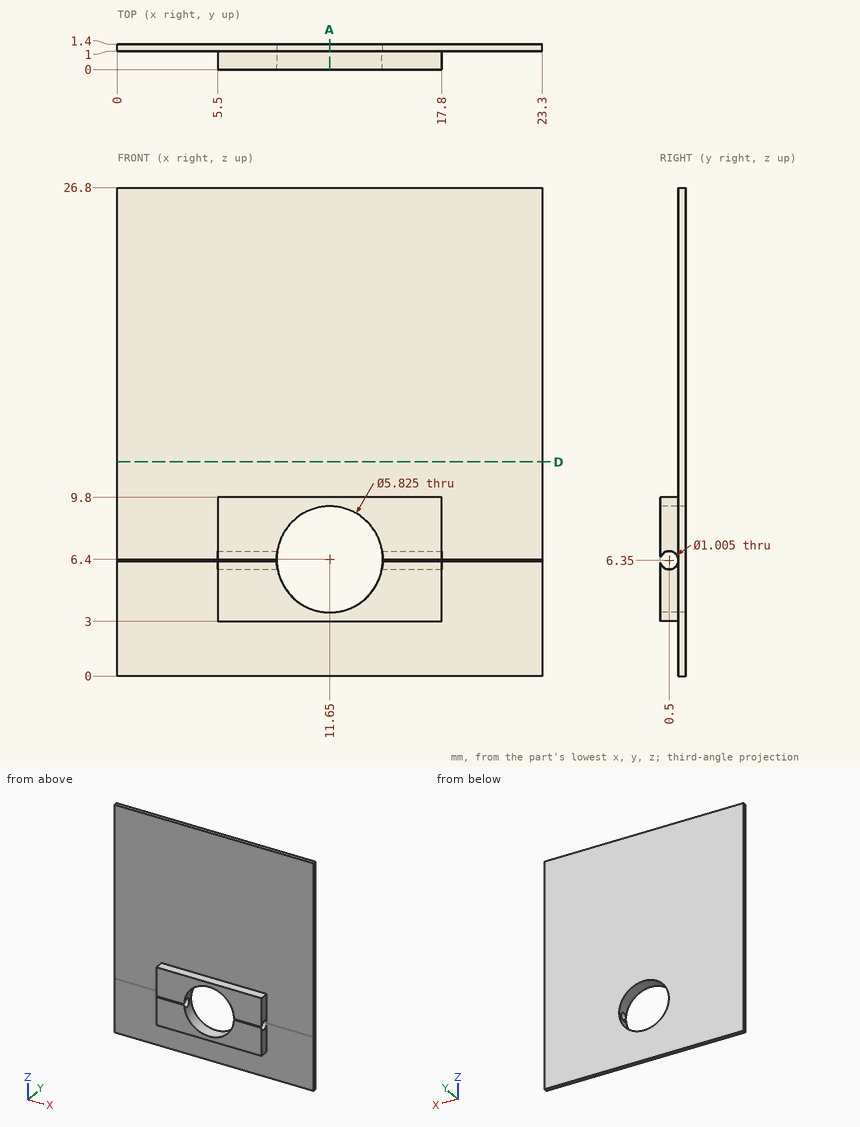
Print and shaded views of the part. All mm, measured from the part's lowest x, y and z. Coordinates: 2 decimals unless noted, no trailing zeros. Loops run counter-clockwise (first coordinate to the right, second up) from the corner with the lowest first, then second, coordinate; pieces in that order, holes last. Notation, with made-up numbers: M -3.75,11.25 L 49.25,11.25 A28 ccw 49.25,47.25 Z; hole C 86,86 d11. An arc over 180 degrees is marked long. Use a Markdown table: item, result. Add a question column.
Q1. Pin check, flat tips, straight feed: P1, Ø0.8, axis at x = 10, y = 0.5, coming from the -Z side; P2, Ø0.5, axis at y = 0.5, z = 4, coming from the -X side; P3, Ø0.8, axis at y = 0.5, z = 8, coming from the +X side; P4, Ø1.9, axis at x = 13, z = 2.5, coming from the -Y side. Stop position of each tip, or through.
Q2. Probe L1, parallel to Z at x = 6.25, y = 0.5; L2, parallel to Z at x = 11.65, y = 0.4; L3, parallel to Y at x = 19, z = 16.25. List the from-to ranges inside material, lowest first.
Q3. Cut at A-A (x = 11.65). Write the cut outline in (y, z).
Q4. Cut at D-D (z = 11.75). Write the cut outline in (x, y).
Worked out:
| question | item | result |
|---|---|---|
| 1 | P1 | stops at z = 3 |
| 1 | P2 | stops at x = 5.5 |
| 1 | P3 | stops at x = 17.8 |
| 1 | P4 | stops at y = 0 |
| 2 | L1 | z = 3 to 5.85, 6.85 to 9.8 |
| 2 | L2 | z = 3 to 3.49, 9.31 to 9.8 |
| 2 | L3 | y = 1 to 1.4 |
| 3 | outline | M 0,3 L 1,3 L 1,0 L 1.4,0 L 1.4,3.49 L 0,3.49 Z; M 0,9.31 L 1.4,9.31 L 1.4,26.8 L 1,26.8 L 1,9.8 L 0,9.8 Z |
| 4 | outline | M 0,1 L 23.3,1 L 23.3,1.4 L 0,1.4 Z |
